from build123d import *

# Parameters (mm, degrees)
SKETCH1_W           = 50
SKETCH1_H           = 60
BOSS_EXTRUDE1_DEPTH = 10
SKETCH2_R           = 1.5
CUT_EXTRUDE1_DEPTH  = 6
CUT_EXTRUDE2_REACH  = 41.509
SKETCH3_R           = 3
SKETCH5_W           = 25
SKETCH5_H           = 6
BOSS_EXTRUDE3_DEPTH = 42
CUT_EXTRUDE3_REACH  = 85.241
SKETCH6_W           = 22
SKETCH6_H           = 19.25
SKETCH7_R           = 1
CUT_EXTRUDE4_DEPTH  = 2.5
CUT_EXTRUDE5_REACH  = 82.754
SKETCH8_R           = 2
BOSS_EXTRUDE4_DEPTH = 5
CHAMFER1_SIZE       = 7.5
CHAMFER2_SIZE       = 10
CHAMFER4_SIZE       = 6.5
CHAMFER5_SIZE       = 4
CHAMFER6_SIZE       = 4
CHAMFER7_SIZE       = 2
CUT_EXTRUDE6_REACH  = 85.241
SKETCH10_R          = 3.1
CHAMFER8_SIZE       = 1


# Some blends are built 0.0001 mm under size
with BuildPart() as part:
    # Sketch1 → Boss-Extrude1 (new body)
    with BuildSketch(Plane(origin=(0, 0, 0), x_dir=(1, 0, 0), z_dir=(0, 1, 0))):
        Rectangle(SKETCH1_W, SKETCH1_H)
    extrude(amount=BOSS_EXTRUDE1_DEPTH)

    # Sketch2 → Cut-Extrude1 (cut)
    with BuildSketch(Plane(origin=(0, 0, 0), x_dir=(1, 0, 0), z_dir=(0, 1, 0))):
        with Locations(Location((-21, 7.7, 0), (0, 0, 270))):
            Circle(SKETCH2_R)
        with Locations(Location((-21, -23, 0), (0, 0, 270))):
            Circle(SKETCH2_R)
        with Locations(Location((21, 7.7, 0), (0, 0, 270))):
            Circle(SKETCH2_R)
        with Locations(Location((21, -23, 0), (0, 0, 270))):
            Circle(SKETCH2_R)
    extrude(amount=CUT_EXTRUDE1_DEPTH, mode=Mode.SUBTRACT)

    # Sketch3 → Cut-Extrude2 (cut, up to next)
    with BuildSketch(Plane.XZ.offset(-6), mode=Mode.PRIVATE) as cut_extrude2_sk1:
        with Locations(Location((-21, 23, 0), (0, 0, 270))):
            Circle(SKETCH3_R)
    cut_extrude2_tool1 = extrude(cut_extrude2_sk1.sketch, amount=-CUT_EXTRUDE2_REACH, mode=Mode.PRIVATE) & part.part
    # Sketch3 → Cut-Extrude2 (cut, up to next)
    with BuildSketch(Plane.XZ.offset(-6), mode=Mode.PRIVATE) as cut_extrude2_sk2:
        with Locations(Location((21, 23, 0), (0, 0, 270))):
            Circle(SKETCH3_R)
    cut_extrude2_tool2 = extrude(cut_extrude2_sk2.sketch, amount=-CUT_EXTRUDE2_REACH, mode=Mode.PRIVATE) & part.part
    # Sketch3 → Cut-Extrude2 (cut, up to next)
    with BuildSketch(Plane.XZ.offset(-6), mode=Mode.PRIVATE) as cut_extrude2_sk3:
        with Locations(Location((21, -7.7, 0), (0, 0, 270))):
            Circle(SKETCH3_R)
    cut_extrude2_tool3 = extrude(cut_extrude2_sk3.sketch, amount=-CUT_EXTRUDE2_REACH, mode=Mode.PRIVATE) & part.part
    # Sketch3 → Cut-Extrude2 (cut, up to next)
    with BuildSketch(Plane.XZ.offset(-6), mode=Mode.PRIVATE) as cut_extrude2_sk4:
        with Locations(Location((-21, -7.7, 0), (0, 0, 270))):
            Circle(SKETCH3_R)
    cut_extrude2_tool4 = extrude(cut_extrude2_sk4.sketch, amount=-CUT_EXTRUDE2_REACH, mode=Mode.PRIVATE) & part.part
    add(cut_extrude2_tool1.solids().sort_by_distance((-21, 6, 23))[0], mode=Mode.SUBTRACT)
    add(cut_extrude2_tool2.solids().sort_by_distance((21, 6, 23))[0], mode=Mode.SUBTRACT)
    add(cut_extrude2_tool3.solids().sort_by_distance((21, 6, -7.7))[0], mode=Mode.SUBTRACT)
    add(cut_extrude2_tool4.solids().sort_by_distance((-21, 6, -7.7))[0], mode=Mode.SUBTRACT)

    # Sketch5 → Boss-Extrude3 (add)
    with BuildSketch(Plane(origin=(0, 10, 0), x_dir=(1, 0, 0), z_dir=(0, 1, 0))):
        with Locations((0, 27)):
            Rectangle(SKETCH5_W, SKETCH5_H)
    extrude(amount=BOSS_EXTRUDE3_DEPTH)

    # Sketch6 → Cut-Extrude3 (cut, up to next)
    with BuildSketch(Plane(origin=(0, 0, -30), x_dir=(-1, 0, 0), z_dir=(0, 0, -1)), mode=Mode.PRIVATE) as cut_extrude3_sk1:
        with Locations((0, 24.625)):
            Rectangle(SKETCH6_W, SKETCH6_H)
    cut_extrude3_tool1 = extrude(cut_extrude3_sk1.sketch, amount=-CUT_EXTRUDE3_REACH, mode=Mode.PRIVATE) & part.part
    add(cut_extrude3_tool1.solids().sort_by_distance((0, 24.625, -30))[0], mode=Mode.SUBTRACT)

    # Sketch7 → Cut-Extrude4 (cut)
    with BuildSketch(Plane.XY.offset(-24)):
        with Locations((10.25, 12.25)):
            Circle(SKETCH7_R)
        with Locations((-10.25, 12.25)):
            Circle(SKETCH7_R)
        with Locations((-10.25, 36.7)):
            Circle(SKETCH7_R)
        with Locations((10.25, 36.7)):
            Circle(SKETCH7_R)
    extrude(amount=-CUT_EXTRUDE4_DEPTH, mode=Mode.SUBTRACT)

    # Sketch8 → Cut-Extrude5 (cut, up to next)
    with BuildSketch(Plane.XY.offset(-26.5), mode=Mode.PRIVATE) as cut_extrude5_sk1:
        with Locations((-10.25, 36.7)):
            Circle(SKETCH8_R)
    cut_extrude5_tool1 = extrude(cut_extrude5_sk1.sketch, amount=-CUT_EXTRUDE5_REACH, mode=Mode.PRIVATE) & part.part
    # Sketch8 → Cut-Extrude5 (cut, up to next)
    with BuildSketch(Plane.XY.offset(-26.5), mode=Mode.PRIVATE) as cut_extrude5_sk2:
        with Locations((10.25, 36.7)):
            Circle(SKETCH8_R)
    cut_extrude5_tool2 = extrude(cut_extrude5_sk2.sketch, amount=-CUT_EXTRUDE5_REACH, mode=Mode.PRIVATE) & part.part
    # Sketch8 → Cut-Extrude5 (cut, up to next)
    with BuildSketch(Plane.XY.offset(-26.5), mode=Mode.PRIVATE) as cut_extrude5_sk3:
        with Locations((10.25, 12.25)):
            Circle(SKETCH8_R)
    cut_extrude5_tool3 = extrude(cut_extrude5_sk3.sketch, amount=-CUT_EXTRUDE5_REACH, mode=Mode.PRIVATE) & part.part
    # Sketch8 → Cut-Extrude5 (cut, up to next)
    with BuildSketch(Plane.XY.offset(-26.5), mode=Mode.PRIVATE) as cut_extrude5_sk4:
        with Locations((-10.25, 12.25)):
            Circle(SKETCH8_R)
    cut_extrude5_tool4 = extrude(cut_extrude5_sk4.sketch, amount=-CUT_EXTRUDE5_REACH, mode=Mode.PRIVATE) & part.part
    add(cut_extrude5_tool1.solids().sort_by_distance((-10.25, 36.7, -26.5))[0], mode=Mode.SUBTRACT)
    add(cut_extrude5_tool2.solids().sort_by_distance((10.25, 36.7, -26.5))[0], mode=Mode.SUBTRACT)
    add(cut_extrude5_tool3.solids().sort_by_distance((10.25, 12.25, -26.5))[0], mode=Mode.SUBTRACT)
    add(cut_extrude5_tool4.solids().sort_by_distance((-10.25, 12.25, -26.5))[0], mode=Mode.SUBTRACT)

    # Sketch9 → Boss-Extrude4 (add)
    with BuildSketch(Plane(origin=(12.5, 0, 0), x_dir=(0, 0, -1), z_dir=(1, 0, 0))):
        Polygon((30, 52), (24, 52), (-18, 10), (30, 10), align=None)
    boss_extrude4 = extrude(amount=BOSS_EXTRUDE4_DEPTH)

    # Mirror1: Boss-Extrude4 across plane
    add(boss_extrude4.mirror(Plane(origin=(0, 0, 0), x_dir=(0, 0, 1), z_dir=(1, 0, 0))))

    # Chamfer1
    # the kernel refuses this chamfer: 7.5 mm, written as the material it adds along each edge
    with BuildSketch(Plane(origin=(17.5, 10, 37.28762241), x_dir=(-0.02749587661058632, 0.9996219169112968, 0), z_dir=(0, 0, -1))) as chamfer1_piece_1_section:
        Polygon((CHAMFER1_SIZE * 0.999621916911, CHAMFER1_SIZE * 0.0274958766106), (-CHAMFER1_SIZE * 0.0274958766106, CHAMFER1_SIZE * 0.999621916911), (0, 0), align=None)
    chamfer1_piece_1 = extrude(amount=67.28762241, mode=Mode.PRIVATE)
    chamfer1_piece_1 = split(chamfer1_piece_1, bisect_by=Plane(origin=(18.496268946, 33.174911168, -5.174911168), z_dir=(0, -0.7071067811865462, -0.7071067811865489)), keep=Keep.TOP, mode=Mode.PRIVATE)
    chamfer1_piece_1 = chamfer1_piece_1 - Plane(origin=(21, 16.349822336, -7.7), x_dir=(0, 0, -1), z_dir=(0, -1, 0)) * Cylinder(3, 165, mode=Mode.PRIVATE)
    chamfer1_piece_1 = split(chamfer1_piece_1, bisect_by=Plane(origin=(25, 16.349822336, -22), z_dir=(-1, 0, 0)), keep=Keep.TOP, mode=Mode.PRIVATE)
    add(chamfer1_piece_1)
    with BuildSketch(Plane(origin=(-17.5, 10, 37.28762241), x_dir=(0.02749587661058632, 0.9996219169112968, 0), z_dir=(0, 0, -1))) as chamfer1_piece_2_section:
        Polygon((CHAMFER1_SIZE * 0.999621916911, -CHAMFER1_SIZE * 0.0274958766106), (-CHAMFER1_SIZE * 0.0274958766106, -CHAMFER1_SIZE * 0.999621916911), (0, 0), align=None)
    chamfer1_piece_2 = extrude(amount=67.28762241, mode=Mode.PRIVATE)
    chamfer1_piece_2 = split(chamfer1_piece_2, bisect_by=Plane(origin=(-18.49626887, 33.174911131, -5.174911131), z_dir=(0, -0.7071067811865462, -0.7071067811865489)), keep=Keep.TOP, mode=Mode.PRIVATE)
    chamfer1_piece_2 = chamfer1_piece_2 - Plane(origin=(-21, 16.349822261, -7.7), x_dir=(0, 0, -1), z_dir=(0, -1, 0)) * Cylinder(3, 165, mode=Mode.PRIVATE)
    chamfer1_piece_2 = split(chamfer1_piece_2, bisect_by=Plane(origin=(-25, 16.349822261, -22), z_dir=(1, 0, 0)), keep=Keep.TOP, mode=Mode.PRIVATE)
    add(chamfer1_piece_2)

    # Chamfer2
    chamfer2_edges = [part.edges().sort_by_distance(p)[0] for p in [
        (-25, 5, -30),
        (25, 5, -30),
    ]]
    chamfer(chamfer2_edges, length=CHAMFER2_SIZE)

    # Chamfer4
    chamfer4_edges = [part.edges().sort_by_distance(p)[0] for p in [
        (0, 0, -30),
    ]]
    chamfer(chamfer4_edges, length=CHAMFER4_SIZE)

    # Chamfer5
    chamfer5_edges = [part.edges().sort_by_distance(p)[0] for p in [
        (17.5, 52, -25.75),
        (-17.5, 52, -25.75),
    ]]
    chamfer(chamfer5_edges, length=CHAMFER5_SIZE)

    # Chamfer6
    chamfer6_edges = [part.edges().sort_by_distance(p)[0] for p in [
        (0, 10, 30),
    ]]
    chamfer(chamfer6_edges, length=CHAMFER6_SIZE - 0.0001)  # a hair under: the kernel refuses the full size

    # Chamfer7
    chamfer7_edges = [part.edges().sort_by_distance(p)[0] for p in [
        (-11, 34.25, -27),
        (-11, 15, -27),
        (11, 15, -27),
        (11, 34.25, -27),
    ]]
    chamfer(chamfer7_edges, length=CHAMFER7_SIZE)

    # Sketch10 → Cut-Extrude6 (cut, up to next)
    with BuildSketch(Plane(origin=(0, 0, -30), x_dir=(-1, 0, 0), z_dir=(0, 0, -1)), mode=Mode.PRIVATE) as cut_extrude6_sk1:
        with Locations((0, 45)):
            Circle(SKETCH10_R)
    cut_extrude6_tool1 = extrude(cut_extrude6_sk1.sketch, amount=-CUT_EXTRUDE6_REACH, mode=Mode.PRIVATE) & part.part
    add(cut_extrude6_tool1.solids().sort_by_distance((0, 45, -30))[0], mode=Mode.SUBTRACT)

    # Chamfer8
    chamfer8_edges = [part.edges().sort_by_distance(p)[0] for p in [
        (3.1, 45, -30),
        (3.1, 45, -24),
    ]]
    chamfer(chamfer8_edges, length=CHAMFER8_SIZE)


solid = part.part
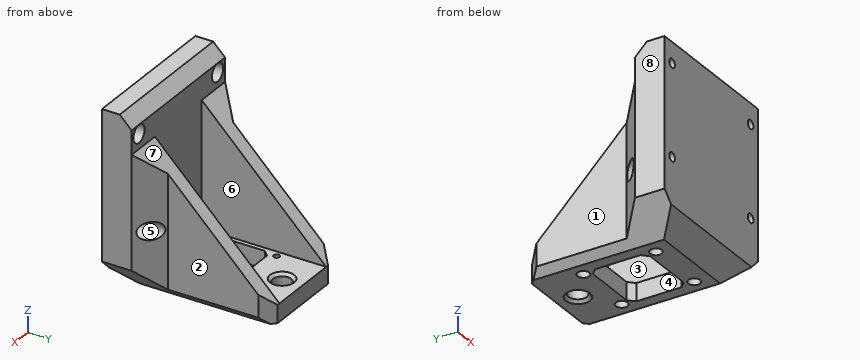
Source: CAD feature listing. Evaluate the final solid. Frame: model axes, mm. Face numbers are marked on the shaded views. A direction names the side the tool comes from. Round coordinates to 2 decimals unless told otherwise and drop trailing zeros. Order: outer loops, then holes, each group sorted by start corner. A loop starts at its lowest first (then second) coordinate and runs counter-clockwise, first axis right, second up. Notation, with made-up numbers: (-1.75, 28) - (3.25, 28) arc R9 ccw to (3.25, 40) - close; hole circle Ø10 at (31, 73). An arc over 180 degrees is marked (long way). Use a Markdown table: item, result. Add a question column.
1. First-contact query: pin 1 (5 mm diameter, centred on y = 17.5, z = -4, fed in from +X); pin 2 (5 mm diameter, centred on x = 21, z = 23, fed in from -Y); pin 3 (24.5 mm diameter, centred on y = 35, z = -11, fed in from -X); pin 4 (15.5 mm diameter, centred on y = 39.5, z = 0.5, fed in from +X). Flat tips, straight axial feed; report the tip coordinate or a pass-through.
2. Line query: probe 1 along X at (y, z) = (12, -25); probe 2 along X at (y, z) = (34.5, -8.5); probe 3 along X at (y, z) = (36, -28). Output: solid intervals per line, ascending.
3. Section query D-D (x = 6.5). Return the cut outline in (y, z).
4. Section query B-B (x = 0). Return the cut outline in (y, z).
5. Set-up query: the marked faces 1, 2, 3, 4 and 5. Return all of +Z, -Z, +X, -X, +Y, -Y with unobstructed straight access to the full face (end or side cutting, diameter ignored); none if empty.
6. Section query A-A (z = 23). Return the cut outline in (x, y).
7. Section query C-C (y = 28). Return the cut outline in (x, z), then the cut area to 3 significant figures.
8. Mould query, pull axis X, two halves, no side actions, for the marked faces 6, 7 and 8. Classes: +X half, -X half, draft (parallel to the pull), parting line (faces both ways), or undercut.
Derived:
| question | item | result |
|---|---|---|
| 1 | pin 1 | x = 20 |
| 1 | pin 2 | y = 0 |
| 1 | pin 3 | x = -17.5 |
| 1 | pin 4 | through |
| 2 | probe 1 | -20 to -11.22, -9.28 to 9.28, 11.22 to 20 |
| 2 | probe 2 | -17.5 to -12.5, 12.5 to 17.5 |
| 2 | probe 3 | -17 to -12.12, -8.38 to 8.38, 12.12 to 17 |
| 3 | outline | (0, -23.5) - (6.5, -30) - (15, -30) - (15, -24) - (10, -24) - (10, 26) - (6, 30) - (0, 30) - close; (34.25, -30) - (52, -30) - (52, -24) - (34.25, -24) - close |
| 4 | outline | (0, -23.5) - (6.5, -30) - (15, -30) - (15, -24) - (10, -24) - (10, 26) - (6, 30) - (0, 30) - close; (34.25, -30) - (40.9, -30) - (41.9, -29) - (41.9, -25) - (40.9, -24) - (34.25, -24) - close; (48.1, -29) - (49.1, -30) - (52, -30) - (52, -24) - (49.1, -24) - (48.1, -25) - close |
| 5 | face 1 | +Z, -Z, -X, +Y |
| 5 | face 2 | +Z, -Z, +X, +Y |
| 5 | face 3 | +Z, +Y |
| 5 | face 4 | +Z, -Z |
| 5 | face 5 | +Y |
| 6 | outline | (-25, 0) - (-22.5, 0) - (-22.5, 6) - (-24, 6) - (-24, 10) - (-25, 10) - close; (-19.5, 0) - (19.5, 0) - (19.5, 6) - (18, 6) - (18, 10) - (-18, 10) - (-18, 6) - (-19.5, 6) - close; (22.5, 0) - (25, 0) - (25, 10) - (24, 10) - (24, 6) - (22.5, 6) - close |
| 7 | outline | (-17.5, -27.5) - (-15, -30) - (-11, -30) - (-11, -24) - (-12.5, -24) - (-12.5, 0) - (-17.5, 0) - close; (11, -30) - (15, -30) - (17.5, -27.5) - (17.5, 0) - (12.5, 0) - (12.5, -24) - (11, -24) - close |
| 7 | area | 312 mm2 |
| 8 | face 6 | undercut |
| 8 | face 7 | draft |
| 8 | face 8 | -X half |
